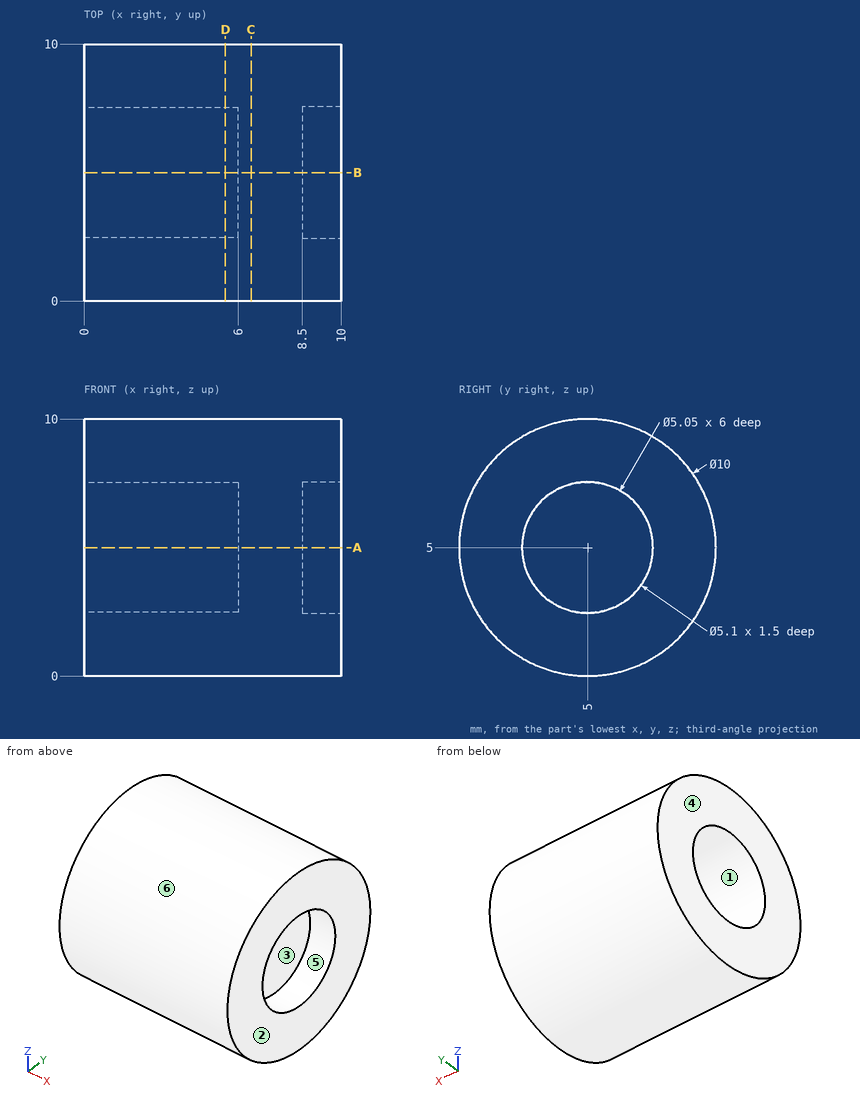
The drawing under review shows one solid part. Ordinate dimensions are in mm from its lowest x, y, z. A direction names the side the tool comes from. Coordinates: 2 decimals unless noted, no trailing zeros. Order: outer loops, then holes, each group sorted by start corner. A loop starts at its lowest first (then second) coordinate and runs counter-clockwise, first axis right, second up. Notation, with made-up numbers: (52.5, 48.25) -> (88.5, 48.25) arc R27 cw to (88.5, 69.25) -> close; hole circle Ø8 at (-31, 27.5). An arc over 180 degrees is marked (long way). One line per item, written item: value.
1) Draft analysis for pull direction Z (two halves, no side actions). For the marked faces 3, 4, 5 and 6, state which applies: +Z half, -Z half, draft (parallel to the pull), parting line (faces both ways), or undercut.
Output values:
face 3: undercut
face 4: draft
face 5: undercut
face 6: parting line
2) Clearance check with flat-ended pins moving along their axes: P1, Ø1.5, axis at y = 6, z = 5, coming from the -X side; P2, Ø1, axis at x = 3.5, z = 3.5, coming from the +Y side; P3, Ø3, axis at x = 2, y = 2, coming from the +Z side. State where each tip first meets the part, or that it passes through.
Output values:
P1: stops at x = 6
P2: stops at y = 9.9
P3: stops at z = 9.77
3) To check wall thickness, follow probe 1 along Z at (x, y) = (8.9, 5); probe 2 along Y at (x, z) = (9, 5.25); probe 3 along Y at (x, z) = (4.25, 7.25). State the ranges of each line that lie inside material, in increasing order. Write a range as [from, to].
Output values:
probe 1: z = [0, 2.45], [7.55, 10]
probe 2: y = [0.01, 2.46], [7.54, 9.99]
probe 3: y = [0.53, 3.85], [6.15, 9.47]
4) Machinability: for the marked faces 1 and 2, which of the approach directions +Z, -Z, +X, -X, +Y, -Y give a long, thin tool a straight path to every point of the face, cutting with its end or side? Answer none if there is none.
Output values:
face 1: -X
face 2: +Z, -Z, +X, +Y, -Y
5) We need section A-A, the plane z = 5. Give the boundary of the cut face in (x, y) (3 decimals), then the cut area to 4 significant figures.
Output values:
outline: (0, 0) -> (10, 0) -> (10, 2.45) -> (8.5, 2.45) -> (8.5, 7.55) -> (10, 7.55) -> (10, 10) -> (0, 10) -> (0, 7.525) -> (6, 7.525) -> (6, 2.475) -> (0, 2.475) -> close
area: 62.05 mm2
6) We need section D-D, the plane x = 5.5. Give the boundary of the cut face in (y, z) (3 decimals).
Output values:
outline: circle Ø10 at (5, 5); hole circle Ø5.05 at (5, 5)
7) We need section C-C, the plane x = 6.5. Give the boundary of the cut face in (y, z), then the cut area to 3 significant figures.
Output values:
outline: circle Ø10 at (5, 5)
area: 78.5 mm2
